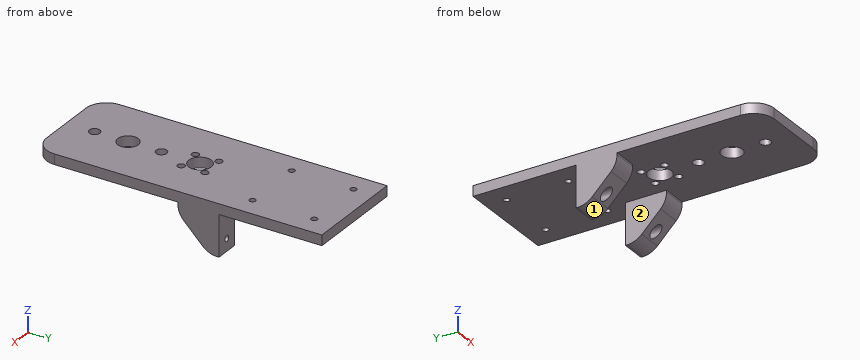
Autodesk Inventor part; units mm, degrees
ref_plane "YZ Plane" through (0, 0, 0) normal (1, 0, 0) x (0, 1, 0)
ref_plane "XZ Plane" through (0, 0, 0) normal (0, 1, 0) x (-1, 0, 0)
ref_plane "XY Plane" through (0, 0, 0) normal (0, 0, 1) x (1, 0, 0)
sketch "Sketch1" plane through (0, 0, 0) normal (0, 0, 1) x (1, 0, 0)
  line L0 (25, 11) -> (-25, 11)
  line L1 (-25, 61) -> (25, 61)
  line L2 (25, 61) -> (25, -39)
  line L3 (25, -39) -> (-25, -39)
  line L4 (-25, -39) -> (-25, 61)
  line L5 (-25, 61) -> (25, -39) construction
  line L6 (25, 61) -> (-25, -39) construction
  line L7 (25, -39) -> (-25, -39)
  line L8 (-25, -39) -> (-25, -89)
  line L9 (-25, -89) -> (25, -89)
  line L10 (25, -89) -> (25, -39)
  point P0 (0, 0)
  point P1 (0, 11)
  dimension "d0" = 50
  dimension "d1" = 100
  dimension "d2" = 50
  dimension "d3" = 50
extrude "Extrusion1" add sketch "Sketch1" along normal blind 5
fillet "Fillet1" radius 10 2 edges at (25, -89, 2.5) (-25, -89, 2.5)
ref_plane "Work Plane1" through (-15, 11, 0) normal (0, -1, 0) x (1, 0, 0)
sketch "Sketch2" plane through (-15, 11, 0) normal (0, -1, 0) x (1, 0, 0)
  line L0 (40, -0.5) -> (-10, -0.5)
  line L1 (-10, -0.5) -> (-10, -3.5)
  line L2 (40, -3.5) -> (-10, -3.5)
  line L3 (40, -0.5) -> (40, -3.5)
  line L4 (-10, -3.5) -> (40, -3.5)
  line L5 (-10, -3.5) -> (-10, -53.5)
  line L6 (-10, -53.5) -> (40, -53.5)
  line L7 (40, -53.5) -> (40, -3.5)
  line L8 (40, -3.5) -> (-10, -3.5)
  ellipse E0 centre (15, -28.5) end of major axis (18.5, -28.5) minor radius 3.5
  line L9 (-10, 0) -> (0, 0)
  line L10 (40, 0) -> (-10, 0)
  line L11 (30, 0) -> (40, 0)
  line L12 (0, 0) -> (30, 0)
  line L13 (25, -0.5) -> (5, -0.5)
  line L14 (5, -0.5) -> (5, -20.5)
  line L15 (25, -20.5) -> (5, -20.5)
  line L16 (25, -0.5) -> (25, -20.5)
  line L17 (40, 0) -> (28, 0)
  line L18 (28, 0) -> (28, -20)
  line L19 (28, -20) -> (40, -20)
  line L20 (40, -20) -> (40, 0)
  line L21 (-10, 0) -> (2, 0)
  line L22 (2, 0) -> (2, -20)
  line L23 (2, -20) -> (-10, -20)
  line L24 (-10, -20) -> (-10, 0)
  point P0 (15, 0)
  dimension "d8" = 12
  dimension "d9" = 20
  dimension "d10" = 12
  dimension "d11" = 20
extrude "Extrusion2" add sketch "Sketch2" along normal blind 20 contours L18 L10 L20 L0 | L0 L3 L2 L18 | L22 L2 L1 L0 | L0 L24 L9 L10 L22 | L2 L7 L19 L18 | L22 L23 L5 L2
chamfer "Chamfer1" distance 15 angle 45 2 edges at (-19, -9, -20) (19, -9, -20)
fillet "Fillet2" radius 10 2 edges at (-19, 6, -20) (-19, -9, -5)
fillet "Fillet3" radius 10 2 edges at (19, -9, -5) (19, 6, -20)
sketch "Sketch3" plane through (0, 0, 5) normal (0, 0, 1) x (1, 0, 0)
  line L0 (25, -79) -> (25, 61)
  line L1 (-25, 61) -> (-25, -79)
  line L2 (25, 61) -> (-25, 61)
  line L3 (-25, 61) -> (-25, 11)
  line L4 (-25, 11) -> (25, 11)
  line L5 (25, 11) -> (25, 61)
  line L6 (-15, 51) -> (15, 51)
  line L7 (15, 51) -> (15, 21)
  line L8 (15, 21) -> (-15, 21)
  line L9 (-15, 21) -> (-15, 51)
  line L10 (-15, 51) -> (15, 21) construction
  line L11 (15, 51) -> (-15, 21) construction
  circle A0 centre (15, 21) radius 1.5
  circle A1 centre (15, 51) radius 1.5
  circle A2 centre (-15, 51) radius 1.5
  circle A3 centre (-15, 21) radius 1.5
  point P0 (0, 0)
  point P1 (0, 36)
  dimension "d19" = 50
  dimension "d20" = 30
  dimension "d21" = 30
  dimension "d22" = 3
  dimension "d23" = 3
  dimension "d24" = 3
  dimension "d25" = 3
extrude "Extrusion3" cut sketch "Sketch3" against normal blind 20 contours L9 A2 L6 | L6 A2 L9 | A1 L7 L6 | L6 L7 A1 | A3 L8 L9 | L9 L8 A3 | A0 L8 L7 | L7 L8 A0
sketch "Sketch4" plane through (-15, 11, 0) normal (0, 1, 0) x (1, 0, 0)
  line L0 (-10, 0) -> (-10, 20)
  line L1 (-10, 20) -> (2, 20)
  line L2 (2, 20) -> (2, 8)
  line L3 (2, 8) -> (-10, 8)
  line L4 (-10, 8) -> (-10, 20)
  circle A0 centre (-4, 14) radius 1.5
  circle A1 centre (34, 14) radius 1.5
  point P0 (15, 0)
  dimension "d28" = 12
  dimension "d29" = 12
  dimension "d30" = 3
  dimension "d33" = 38
extrude "Extrusion4" cut sketch "Sketch4" against normal through all contours A0 | A1
sketch "Sketch5" plane through (-15, -9, 0) normal (0, -1, 0) x (1, 0, 0)
  circle A0 centre (34, -14) radius 1.5
  circle A1 centre (-4, -14) radius 1.5
  circle A2 centre (34, -14) radius 2.5
  circle A3 centre (-4, -14) radius 1.5
  circle A4 centre (-4, -14) radius 2.5
  point P0 (15, 0)
  dimension "d40" = 5
  dimension "d41" = 5
extrude "Extrusion5" cut sketch "Sketch5" against normal blind 15
sketch "Sketch6" plane through (0, 0, 5) normal (0, 0, 1) x (1, 0, 0)
  circle A0 centre (0, -49) radius 5
  line L0 (25, 61) -> (-25, 61)
  circle A1 centre (0, -32.75) radius 2.6
  circle A2 centre (0, -65.25) radius 2.6
  circle A3 centre (0, -14) radius 5.5
  point P0 (0, 0)
  dimension "d44" = 10
  dimension "d45" = 110
  dimension "d46" = 5.2
  dimension "d47" = 5.2
  dimension "d48" = 16.25
  dimension "d49" = 16.25
  dimension "d52" = 11
  dimension "d53" = 75
extrude "Extrusion6" cut sketch "Sketch6" against normal blind 10
sketch "Sketch7" plane through (0, 0, 5) normal (0, 0, 1) x (1, 0, 0)
  circle A0 centre (-5.7947, -8.4844) radius 1.75
  circle A1 centre (-5.5156, -19.7947) radius 1.75
  circle A2 centre (5.7947, -19.5156) radius 1.75
  circle A3 centre (5.5156, -8.2053) radius 1.75
  point P0 (0, 0)
extrude "Extrusion7" cut sketch "Sketch7" against normal through all
sketch "Sketch8" plane through (0, 0, 5) normal (0, 0, 1) x (1, 0, 0)
  line L0 (-25, 61) -> (-25, -79)
  arc A0 (15, -89) -> (25, -79) centre (15, -79) ccw
  line L1 (-25, -79) -> (25, -79)
  circle A1 centre (5.7947, -19.5156) radius 1.75
  circle A2 centre (-5.5156, -19.7947) radius 1.75
  circle A3 centre (5.5156, -8.2053) radius 1.75
  circle A4 centre (-5.7947, -8.4844) radius 1.75
  circle A5 centre (0, -32.75) radius 2.6
  circle A6 centre (0, -49) radius 5
  circle A7 centre (0, -65.25) radius 2.6
  circle A8 centre (0, -14) radius 5.5
  circle A9 centre (-15, 21) radius 1.5
  circle A10 centre (15, 21) radius 1.5
  circle A11 centre (-15, 51) radius 1.5
  circle A12 centre (15, 51) radius 1.5
  arc A13 (-25, -79) -> (-15, -89) centre (-15, -79) ccw
  line L2 (-15, -89) -> (15, -89)
  arc A14 (15, -89) -> (25, -79) centre (15, -79) ccw
  line L3 (25, -79) -> (25, 61)
  line L4 (25, 61) -> (-25, 61)
  line L5 (-25, 61) -> (-25, -79)
  point P0 (0, 0)
extrude "Extrusion8" cut sketch "Sketch8" against normal blind 10 contours L1 A0 L2 A13
fillet "Fillet4" radius 10 2 edges at (25, -79, 2.5) (-25, -79, 2.5)
properties part number "3d mount for linear bearing"
For this review, take the finished solid that the model builds, in its own axes (mm). Face numbers are marked on the shaded views. Round coordinates to 2 decimals unless told otherwise and drop trailing zeros. Order: outer loops, then holes, each group sorted by start corner. A loop starts at its lowest first (then second) coordinate and runs counter-clockwise, first axis right, second up. Notation, with made-up numbers: M 57.25,89.25 L 88.25,89.25 A27 ccw 88.25,123.25 Z; hole C 22.5,13 d7. An arc over 180 degrees is marked long. Write each question's results on one line, items separated by ' | '. Start each with the question number.
1. Add section D-D (z = -6). State the section outline as (x, y) points.
2. Add section A-A (y = -32.75). State the section outline as (x, z) points.
3. Add section B-B (z = -14). State the section outline as (x, y) points, then the cut area to 3 significant figures.
4. To check wall thickness, follow L1, parallel to Y at x = -15, z = 3.2; L2, parallel to Y at x = 0, z = 2.25; L3, parallel to X at y = 51, z = 1.4. State the ranges of each line that lie inside material, in increasing order. Write a range as [from, to].
5. Draft analysis for pull direction Y (two halves, no side actions). For the marked faces 1 and 2, state which applies: pulls with the +Y half, pulls with the -Y half, needs draft (parallel to the pull), parting line crosses it, or undercut.
6. Clearance check with flat-ended pins moving along their axes: pin 1 Ø3 at (x, y) = (0, -32.75) entering from -Z; pin 2 Ø1.5 at (x, z) = (18, -15) entering from -Y; pin 3 Ø4 at (x, z) = (-19, -14) entering from +Y; pin 4 Ø5 at (x, y) = (-14, -5) entering from -Z. State where each tip first meets the part, or that it passes through.
7. Add section C-C (y = 51). State the section outline as (x, z) points.
Output values:
1) outline: M -25,-7.58 L -13,-7.58 L -13,11 L -25,11 Z; M 13,-7.58 L 25,-7.58 L 25,11 L 13,11 Z
2) outline: M -25,0 L -2.6,0 L -2.6,5 L -25,5 Z; M 2.6,0 L 25,0 L 25,5 L 2.6,5 Z
3) outline: M -25,0 L -21.5,0 L -21.5,6 L -20.5,6 L -20.5,11 L -25,11 Z; M -17.5,6 L -16.5,6 L -16.5,0 L -13,0 L -13,11 L -17.5,11 Z; M 13,0 L 16.5,0 L 16.5,6 L 17.5,6 L 17.5,11 L 13,11 Z; M 20.5,6 L 21.5,6 L 21.5,0 L 25,0 L 25,11 L 20.5,11 Z | area: 174 mm^2
4) L1: [-79, 19.5], [22.5, 49.5], [52.5, 61] | L2: [-79, -67.85], [-62.65, -54], [-44, -35.35], [-30.15, -19.5], [-8.5, 61] | L3: [-25, -16.5], [-13.5, 13.5], [16.5, 25]
5) face 1: pulls with the -Y half | face 2: needs draft
6) pin 1: through | pin 2: y = 6 | pin 3: y = 11 | pin 4: z = -11.5
7) outline: M -25,0 L -16.5,0 L -16.5,5 L -25,5 Z; M -13.5,0 L 13.5,0 L 13.5,5 L -13.5,5 Z; M 16.5,0 L 25,0 L 25,5 L 16.5,5 Z
